Source: CAD feature listing. Evaluate the final solid. Frame: model axes, mm. A direction names the side the tool comes from. Give positions to 0.01 mm unless a question says otherwise; leave off trailing zeros. Write each loop counter-clockwise with the first axis right and the second up, starting at its lowest first coordinate (ties: lowest second). Pieces come first, ordered by that corner, then holes. Notation, with made-up numbers: (34, -22) -> (77, -22) arc R18 cw to (77, -2) -> close; hole circle Ø6 at (62, -23.5). An arc over 180 degrees is marked (long way). Answer as a JSON object with one key per item and string values. Group by question number.
Item 1: Section query A-A on x = 63.5. Return the cut outline in (y, z).
Item 2: Ray query, probe 1 along Z at (x, y) = (-63.5, -23); probe 2 along Y at (x, z) = (-57.5, 21.5); probe 3 along X at (y, z) = (-43.5, 10). Return the intervals inside material, ascending. Write a range as from..to.
Item 3: Section query B-B on y = -36.5. Return the cut outline in (x, z).
Item 4: Pull-direction query (X, two-part tool) for faces 1 (the face through (-133.35, -22, -1)), 2 (the face through (-82.53, -31.48, 4.56)), 3 (the face through (-2, -22, -76.2)); classes: pulls with the +X half, pulls with the -X half, needs draft (parallel to the pull), parting line crosses it, or undercut.
Item 5: Access query for faces 4 (the face through (133.35, -22, -1)), 5 (the face through (0, -12.7, 4)). Directions: +Z, -Z, +X, -X, +Y, -Y. A direction counts if a zero-diameter tool reaches every point of the face in a straight line with its end or side. Return the directions, or none.
Item 6: First-contact query: pin 1 Ø23 at (x, z) = (0, 3.73) entering from -Y. Flat tip, straight axial feed; report the tip coordinate or a pass-through.
from build123d import *

# Parameters (mm, degrees)
F0_W     = 266.7
F0_H     = 152.4
F0_R     = 19.05
F1_DEPTH = 50.8
F2_DEPTH = 12.7
F3_R     = 6.35


with BuildPart() as f1:
    # F0 (on Front) → F1 (new body)
    with BuildSketch(Plane.XZ):
        Rectangle(F0_W, F0_H)
        with Locations((-63.5, 3.7267601583)):
            Circle(F0_R, mode=Mode.SUBTRACT)
        with BuildLine():
            ThreePointArc((-19.05, 3.7267601583), (0, 22.7767601583), (19.05, 3.7267601583))
            ThreePointArc((19.05, 3.7267601583), (0, -15.3232398417), (-19.05, 3.7267601583))
        make_face(mode=Mode.SUBTRACT)
        with BuildLine():
            ThreePointArc((82.55, 3.7267601583), (63.5, -15.3232398417), (44.45, 3.7267601583))
            ThreePointArc((44.45, 3.7267601583), (63.5, 22.7767601583), (82.55, 3.7267601583))
        make_face(mode=Mode.SUBTRACT)
    extrude(amount=F1_DEPTH)

    # F0 (on Front) → F2 (join)
    with BuildSketch(Plane.XZ):
        with BuildLine():
            ThreePointArc((-19.05, 3.7267601583), (0, -15.3232398417), (19.05, 3.7267601583))
            ThreePointArc((19.05, 3.7267601583), (0, 22.7767601583), (-19.05, 3.7267601583))
        make_face()
        with Locations((-63.5, 3.7267601583)):
            Circle(F0_R)
        with BuildLine():
            ThreePointArc((82.55, 3.7267601583), (63.5, 22.7767601583), (44.45, 3.7267601583))
            ThreePointArc((44.45, 3.7267601583), (63.5, -15.3232398417), (82.55, 3.7267601583))
        make_face()
    extrude(amount=F2_DEPTH)

    # F3
    f3_edges = [f1.edges().sort_by_distance(p)[0] for p in [
        (-133.35, -50.8, 0),
        (0, -50.8, -76.2),
        (133.35, -50.8, 0),
        (0, -50.8, 76.2),
    ]]
    fillet(f3_edges, radius=F3_R)


solid = f1.part
Worked answers:
{
 "1": {"outline": "(-50.8, -69.85) arc R6.35 ccw to (-44.45, -76.2) -> (0, -76.2) -> (0, 76.2) -> (-44.45, 76.2) arc R6.35 ccw to (-50.8, 69.85) -> (-50.8, 22.78) -> (-12.7, 22.78) -> (-12.7, -15.32) -> (-50.8, -15.32) -> close"},
 "2": {"probe 1": "-76.2..-15.32, 22.78..76.2", "probe 2": "-12.7..0", "probe 3": "-133.35..-81.49, -45.51..-17.99, 17.99..45.51, 81.49..133.35"},
 "3": {"outline": "(-133.35, -76.2) -> (133.35, -76.2) -> (133.35, 76.2) -> (-133.35, 76.2) -> close; hole circle Ø38.1 at (-63.5, 3.73); hole circle Ø38.1 at (0, 3.73); hole circle Ø38.1 at (63.5, 3.73)"},
 "4": {"face 1": "pulls with the -X half", "face 2": "undercut", "face 3": "needs draft"},
 "5": {"face 4": "+Z, -Z, +X, +Y, -Y", "face 5": "-Y"},
 "6": {"pin 1": "y = -12.7"}
}
